from build123d import *

# Parameters (mm, degrees)
SKETCH1_W           = 25.4
SKETCH1_H           = 59.944
BOSS_EXTRUDE1_DEPTH = 50.8
SKETCH2_OUTSIDE_W   = 69.316
SKETCH2_OUTSIDE_H   = 78.46
SKETCH2_OUTSIDE_W_2 = 50.8
SKETCH2_OUTSIDE_H_2 = 59.944
SKETCH2_OUTSIDE_R   = 2.5796875
CUT_EXTRUDE1_DEPTH  = 10.16
CUT_EXTRUDE2_REACH  = 66.219
SKETCH3_R           = 3.302
SKETCH4_R           = 6.35
CUT_EXTRUDE3_DEPTH  = 19.05


with BuildPart() as part:
    # Sketch1 → Boss-Extrude1 (new body)
    with BuildSketch(Plane.XY):
        Rectangle(SKETCH1_W, SKETCH1_H)
    extrude(amount=BOSS_EXTRUDE1_DEPTH)

    # Sketch2 outside → Cut-Extrude1 (cut)
    # profile 1 of 5: a face of its own
    with BuildSketch(Plane(origin=(12.7, 0, 0), x_dir=(0, 0, -1), z_dir=(1, 0, 0))):
        with Locations((-25.4, 0)):
            Rectangle(SKETCH2_OUTSIDE_W, SKETCH2_OUTSIDE_H)
        with Locations((-25.4, 0)):
            Rectangle(SKETCH2_OUTSIDE_W_2, SKETCH2_OUTSIDE_H_2, mode=Mode.SUBTRACT)
    # profile 2 of 5: a face of its own
    with BuildSketch(Plane(origin=(12.7, 0, 0), x_dir=(0, 0, -1), z_dir=(1, 0, 0))):
        with Locations(Location((-19, 22.972, 0), (0, 0, 90))):
            Circle(SKETCH2_OUTSIDE_R)
    # profile 3 of 5: a face of its own
    with BuildSketch(Plane(origin=(12.7, 0, 0), x_dir=(0, 0, -1), z_dir=(1, 0, 0))):
        with Locations(Location((-6, 22.972, 0), (0, 0, 90))):
            Circle(SKETCH2_OUTSIDE_R)
    # profile 4 of 5: a face of its own
    with BuildSketch(Plane(origin=(12.7, 0, 0), x_dir=(0, 0, -1), z_dir=(1, 0, 0))):
        with Locations(Location((-19, -23.028, 0), (0, 0, 90))):
            Circle(SKETCH2_OUTSIDE_R)
    # profile 5 of 5: a face of its own
    with BuildSketch(Plane(origin=(12.7, 0, 0), x_dir=(0, 0, -1), z_dir=(1, 0, 0))):
        with Locations(Location((-6, -23.028, 0), (0, 0, 90))):
            Circle(SKETCH2_OUTSIDE_R)
    extrude(amount=-CUT_EXTRUDE1_DEPTH, mode=Mode.SUBTRACT)

    # Sketch3 → Cut-Extrude2 (cut, up to next)
    with BuildSketch(Plane(origin=(12.7, 0, 0), x_dir=(0, 0, -1), z_dir=(1, 0, 0)), mode=Mode.PRIVATE) as cut_extrude2_sk1:
        with Locations(Location((-36.743794207, 12.573, 0), (0, 0, 90))):
            Circle(SKETCH3_R)
    cut_extrude2_tool1 = extrude(cut_extrude2_sk1.sketch, amount=-CUT_EXTRUDE2_REACH, mode=Mode.PRIVATE) & part.part
    # Sketch3 → Cut-Extrude2 (cut, up to next)
    with BuildSketch(Plane(origin=(12.7, 0, 0), x_dir=(0, 0, -1), z_dir=(1, 0, 0)), mode=Mode.PRIVATE) as cut_extrude2_sk2:
        with Locations(Location((-36.743794207, -12.573, 0), (0, 0, 90))):
            Circle(SKETCH3_R)
    cut_extrude2_tool2 = extrude(cut_extrude2_sk2.sketch, amount=-CUT_EXTRUDE2_REACH, mode=Mode.PRIVATE) & part.part
    add(cut_extrude2_tool1.solids().sort_by_distance((12.7, 12.573, 36.743794))[0], mode=Mode.SUBTRACT)
    add(cut_extrude2_tool2.solids().sort_by_distance((12.7, -12.573, 36.743794))[0], mode=Mode.SUBTRACT)

    # Sketch4 → Cut-Extrude3 (cut)
    with BuildSketch(Plane(origin=(12.7, 0, 0), x_dir=(0, 0, -1), z_dir=(1, 0, 0))):
        with Locations(Location((-36.743794207, 12.573, 0), (0, 0, 90))):
            Circle(SKETCH4_R)
        with Locations(Location((-36.743794207, -12.573, 0), (0, 0, 90))):
            Circle(SKETCH4_R)
    extrude(amount=-CUT_EXTRUDE3_DEPTH, mode=Mode.SUBTRACT)


solid = part.part
For this review, take the finished solid that the model builds, in its own axes (mm). A direction names the side the tool comes from. Give positions to 0.01 mm unless a question says otherwise; leave off trailing zeros. Order: outer loops, then holes, each group sorted by start corner. A loop starts at its lowest first (then second) coordinate and runs counter-clockwise, first axis right, second up. Notation, with made-up numbers: (8.5, -16) - (62.5, -16) arc R25 cw to (62.5, 7) - close; hole circle Ø5 at (38, 52.25). An arc over 180 degrees is marked (long way). Answer as a JSON object with one key per item and string values. Group by question number.
Item 1: Draft analysis for pull direction Z (two halves, no side actions). For faces 3 (the cylindrical face through (3.31, 11.75, 43.04)), 4 (the flat face through (0, 0, 0)), 5 (the flat face through (0, -29.972, 25)), 6 (the flat face through (0, 0, 50.8)), state which applies: pulls with the +Z half, pulls with the -Z half, needs draft (parallel to the pull), parting line crosses it, or undercut.
Item 2: Clearance check with flat-ended pins moving along their axes: pin 1 Ø6.5 at (y, z) = (22.972, 19) entering from +X; pin 2 Ø6 at (y, z) = (12.57, 36.74) entering from -X; pin 3 Ø6.5 at (y, z) = (-14.5, 37) entering from +X; pin 4 Ø1.5 at (y, z) = (-23, 19) entering from +X. State where each tip first meets the part, or that it passes through.
Item 3: Take a section at A-A on y = -12. Give the boundary of the cut face in (x, z).
Item 4: Take a section at C-C on x = -9.5. Give the boundary of the cut face in (y, z) (3 decimals), and give its area (3 significant figures).
Item 5: Machinability: for faces 1 (the cylindrical face through (-9.48, -13.29, 33.52)), 2 (the flat face through (2.54, -23, 19)), which of the approach directions +Z, -Z, +X, -X, +Y, -Y give a long, thin tool a straight path to every point of the face, cutting with its end or side? Answer none if there is none.
Item 6: Wall thickness on line 1 along Y through (x, z) = (8, 18.5); line 2 along X through (y, z) = (22, 6.5); line 3 along Z through (x, y) = (10, 23.5): over which ranges is each line inside the solid? List them lowest first.
Item 7: Take a section at B-B on z = 19. Give the boundary of the cut face in (x, y).
Item 8: Take a section at D-D on y = 8.5. Give the boundary of the cut face in (x, z).
Reported:
{
 "1": {"face 3": "undercut", "face 4": "pulls with the -Z half", "face 5": "needs draft", "face 6": "pulls with the +Z half"},
 "2": {"pin 1": "x = 12.7", "pin 2": "through", "pin 3": "x = -6.35", "pin 4": "x = 2.54"},
 "3": {"outline": "(-12.7, 0) - (12.7, 0) - (12.7, 30.42) - (-6.35, 30.42) - (-6.35, 33.49) - (-12.7, 33.49) - close; (-12.7, 40) - (-6.35, 40) - (-6.35, 43.07) - (12.7, 43.07) - (12.7, 50.8) - (-12.7, 50.8) - close"},
 "4": {"outline": "(-29.972, 0) - (29.972, 0) - (29.972, 50.8) - (-29.972, 50.8) - close; hole circle Ø6.604 at (-12.573, 36.744); hole circle Ø6.604 at (12.573, 36.744)", "area": "2,980 mm^2"},
 "5": {"face 1": "+X, -X", "face 2": "+X"},
 "6": {"line 1": "-29.97 to -25.56, -20.5 to 20.44, 25.5 to 29.97", "line 2": "-12.7 to 2.54", "line 3": "0 to 3.47, 8.53 to 16.47, 21.53 to 50.8"},
 "7": {"outline": "(-12.7, -29.97) - (12.7, -29.97) - (12.7, -25.61) - (2.54, -25.61) - (2.54, -20.45) - (12.7, -20.45) - (12.7, 20.39) - (2.54, 20.39) - (2.54, 25.55) - (12.7, 25.55) - (12.7, 29.97) - (-12.7, 29.97) - close"},
 "8": {"outline": "(-12.7, 0) - (12.7, 0) - (12.7, 31.87) - (-6.35, 31.87) - (-6.35, 41.62) - (12.7, 41.62) - (12.7, 50.8) - (-12.7, 50.8) - close"}
}
